from build123d import *

# Parameters (mm, degrees)
F1_DEPTH = 19.05
F3_DEPTH = 76.2


# Not quite as in the source:
# - a feature names something its author has since deleted; it is built from what else it names


with BuildPart() as f1:
    # F0 (on Top) → F1 (new body)
    with BuildSketch(Plane.XY):
        with BuildLine():
            Line((533.4, 317.5), (-533.4, 317.5))
            ThreePointArc((-533.4, 317.5), (-569.3210244843, 302.6210244843), (-584.2, 266.7))
            Line((-584.2, 266.7), (-584.2, -266.7))
            ThreePointArc((-584.2, -266.7), (-569.3210244843, -302.6210244843), (-533.4, -317.5))
            Line((-533.4, -317.5), (533.4, -317.5))
            ThreePointArc((533.4, -317.5), (569.3210244843, -302.6210244843), (584.2, -266.7))
            Line((584.2, -266.7), (584.2, 266.7))
            ThreePointArc((584.2, 266.7), (569.3210244843, 302.6210244843), (533.4, 317.5))
        make_face()
    extrude(amount=F1_DEPTH)

    # F2 (on face) → F3 (join)
    with BuildSketch(Plane.XY.offset(19.05)):
        with BuildLine():
            ThreePointArc((584.2, 266.7), (569.3210244843, 302.6210244843), (533.4, 317.5))
            Line((533.4, 317.5), (-533.4, 317.5))
            ThreePointArc((-533.4, 317.5), (-569.3210244843, 302.6210244843), (-584.2, 266.7))
            Line((-584.2, 266.7), (-584.2, -266.7))
            ThreePointArc((-584.2, -266.7), (-569.3210244843, -302.6210244843), (-533.4, -317.5))
            Line((-533.4, -317.5), (533.4, -317.5))
            ThreePointArc((533.4, -317.5), (569.3210244843, -302.6210244843), (584.2, -266.7))
            Line((584.2, -266.7), (584.2, 266.7))
        make_face()
        with BuildLine():
            Line((-571.5, -266.7), (-571.5, 266.7))
            ThreePointArc((-571.5, 266.7), (-560.3407683632, 293.6407683632), (-533.4, 304.8))
            Line((-533.4, 304.8), (533.4, 304.8))
            ThreePointArc((533.4, 304.8), (560.3407683632, 293.6407683632), (571.5, 266.7))
            Line((571.5, 266.7), (571.5, -266.7))
            ThreePointArc((571.5, -266.7), (560.3407683632, -293.6407683632), (533.4, -304.8))
            Line((533.4, -304.8), (-533.4, -304.8))
            ThreePointArc((-533.4, -304.8), (-560.3407683632, -293.6407683632), (-571.5, -266.7))
        make_face(mode=Mode.SUBTRACT)
    extrude(amount=F3_DEPTH)


solid = f1.part
The model under review builds one solid part; all positions refer to its coordinate system, in mm. A direction names the side the tool comes from. Round coordinates to 2 decimals unless told otherwise and drop trailing zeros. Loops run counter-clockwise (first coordinate to the right, second up) from the corner with the lowest first, then second, coordinate; pieces in that order, holes last. Notation, with made-up numbers: (41.5, -35.5) -> (68.5, -35.5) arc R13 ccw to (68.5, -30.5) -> close; hole circle Ø2 at (78.5, 77). An arc over 180 degrees is marked (long way). Return JSON: item names as keys, results as strings.
(1) For line 1 (X direction, y = 112.5, z = 23); line 2 (Y direction, x = -209, z = 57.5); line 3 (Z direction, x = 344.5, y = 159.5), list the stretches that pass through material, from the lowest coordinate up.
Solved:
{"line 1": "-584.2 to -571.5, 571.5 to 584.2", "line 2": "-317.5 to -304.8, 304.8 to 317.5", "line 3": "0 to 19.05"}
(2) Add section B-B on x = 52. Write out the cut boundary in (y, z), plus the area to 3 significant figures.
Solved:
{"outline": "(-317.5, 0) -> (317.5, 0) -> (317.5, 95.25) -> (304.8, 95.25) -> (304.8, 19.05) -> (-304.8, 19.05) -> (-304.8, 95.25) -> (-317.5, 95.25) -> close", "area": "14,000 mm2"}
(3) Add section C-C on y = 11. Write out the cut boundary in (x, z), plus the area to 3 significant figures.
Solved:
{"outline": "(-584.2, 0) -> (584.2, 0) -> (584.2, 95.25) -> (571.5, 95.25) -> (571.5, 19.05) -> (-571.5, 19.05) -> (-571.5, 95.25) -> (-584.2, 95.25) -> close", "area": "24,200 mm2"}
(4) The part is to be moulded in two halves that separate along X. For faces 3 (the flat face through (-7, 304.8, 57)), 4 (the cylindrical face through (560.04, 293.94, 56.62)), 5 (the cylindrical face through (-568.924, 303.014, 46.958)), 6 (the cylindrical face through (568.924, -303.014, 46.958)), say which applies: released by +X, released by -X, zero draft, split by the parting line, or undercut.
Solved:
{"face 3": "undercut", "face 4": "undercut", "face 5": "released by -X", "face 6": "released by +X"}
(5) For faces 1 (the cylindrical face through (569.714, 302.224, 46.958)), 2 (the cylindrical face through (-560.04, -293.94, 56.62)), list the 3-axis set-ups (+Z, -Z, +X, -X, +Y, -Y) from which the entire face can be reached by the end or side of a thin tool; tool diameter is ignored.
Solved:
{"face 1": "+Z, -Z, +X, +Y", "face 2": "+Z"}
(6) For pin 1 (4 mm diameter, centred on x = 407.5, y = 174.5, fed in from +Z), flat-tipped, find the tip position at first contact; note if it passes through.
Solved:
{"pin 1": "z = 19.05"}
(7) Add section A-A on z = 57. Write out the cut boundary in (x, y), plus the area to 3 significant figures.
Solved:
{"outline": "(-584.2, -266.7) arc R50.8 ccw to (-533.4, -317.5) -> (533.4, -317.5) arc R50.8 ccw to (584.2, -266.7) -> (584.2, 266.7) arc R50.8 ccw to (533.4, 317.5) -> (-533.4, 317.5) arc R50.8 ccw to (-584.2, 266.7) -> close; hole (-571.5, -266.7) arc R38.1 ccw to (-533.4, -304.8) -> (533.4, -304.8) arc R38.1 ccw to (571.5, -266.7) -> (571.5, 266.7) arc R38.1 ccw to (533.4, 304.8) -> (-533.4, 304.8) arc R38.1 ccw to (-571.5, 266.7) -> close", "area": "44,200 mm2"}
